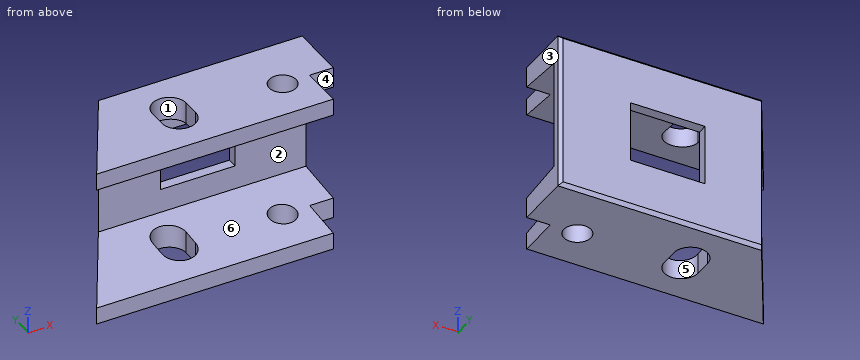
```python
from build123d import *

# Parameters (mm, degrees)
SKETCH1_R           = 4
BOSS_EXTRUDE1_DEPTH = 23.5
CUT_EXTRUDE1_REACH  = 87.914
CUT_EXTRUDE2_REACH  = 58.712
SKETCH3_W           = 22
SKETCH3_H           = 18
CHAMFER1_SIZE       = 1


with BuildPart() as part:
    # Sketch1 → Boss-Extrude1 (new, symmetric)
    with BuildSketch(Plane.XY):
        Polygon((-35, 0), (35, 0), (35, 12.5), (42, 12.5), (42, 30), (-17.679491924, 30), align=None)
        with Locations((27, 12.5)):
            Circle(SKETCH1_R, mode=Mode.SUBTRACT)
        with BuildLine():
            Line((-9, 12), (-9, 17))
            ThreePointArc((-9, 17), (-4, 22), (1, 17))
            Line((1, 17), (1, 12))
            ThreePointArc((1, 12), (-4, 7), (-9, 12))
        make_face(mode=Mode.SUBTRACT)
    extrude(amount=BOSS_EXTRUDE1_DEPTH, both=True)

    # Sketch2 → Cut-Extrude1 (cut, up to next)
    with BuildSketch(Plane(origin=(42, 0, 0), x_dir=(0, 0, -1), z_dir=(1, 0, 0)), mode=Mode.PRIVATE) as cut_extrude1_sk1:
        Polygon((-18.5, 0), (18.5, 0), (16.137806085, 27), (-16.137806085, 27), align=None)
    cut_extrude1_tool1 = extrude(cut_extrude1_sk1.sketch, amount=-CUT_EXTRUDE1_REACH, mode=Mode.PRIVATE) & part.part
    add(cut_extrude1_tool1.solids().sort_by_distance((42, 13.193114, 0))[0], mode=Mode.SUBTRACT)

    # Sketch3 → Cut-Extrude2 (cut, up to next)
    with BuildSketch(Plane(origin=(0, 30, 0), x_dir=(1, 0, 0), z_dir=(0, 1, 0)), mode=Mode.PRIVATE) as cut_extrude2_sk1:
        with Locations((10, 0)):
            Rectangle(SKETCH3_W, SKETCH3_H)
    cut_extrude2_tool1 = extrude(cut_extrude2_sk1.sketch, amount=-CUT_EXTRUDE2_REACH, mode=Mode.PRIVATE) & part.part
    add(cut_extrude2_tool1.solids().sort_by_distance((10, 30, 0))[0], mode=Mode.SUBTRACT)

    # Chamfer1
    chamfer1_edges = [part.edges().sort_by_distance(p)[0] for p in [
        (42, 30, 0),
        (12.160254038, 30, 23.5),
        (12.160254038, 30, -23.5),
    ]]
    chamfer(chamfer1_edges, length=CHAMFER1_SIZE)


solid = part.part
```
For this review, take the finished solid that the model builds, in its own axes (mm). Face numbers are marked on the shaded views. A direction names the side the tool comes from. Round coordinates to 2 decimals unless told otherwise and drop trailing zeros. Loops run counter-clockwise (first coordinate to the right, second up) from the corner with the lowest first, then second, coordinate; pieces in that order, holes last.
(1) We need section D-D (x = 27). Give the boundary of the cut face in (y, z).
Returned:
outline: (0, -23.5) - (8.5, -23.5) - (8.5, -17.76) - (0, -18.5) - close; (0, 18.5) - (8.5, 17.76) - (8.5, 23.5) - (0, 23.5) - close; (16.5, -23.5) - (29, -23.5) - (30, -22.5) - (30, 22.5) - (29, 23.5) - (16.5, 23.5) - (16.5, 17.06) - (27, 16.14) - (27, -16.14) - (16.5, -17.06) - close
(2) Mouldability with a two-part tool opening along Y and no side actions: class the marked faces 1, 2 and 3 as released by +Y, released by -Y, zero draft, split by the parting line, or undercut.
Returned:
face 1: undercut
face 2: released by -Y
face 3: zero draft
(3) Tool access review of the marked faces 4, 5 and 6: name each direction out of +Z, -Z, +X, -X, +Y, -Y from which nothing blocks a thin tool from reaching the whole face with its end or side.
Returned:
face 4: +Z, -Z, +X, -Y
face 5: +Z, -Z
face 6: +X, -X, -Y
(4) Clearance check with flat-ended pins moving along their axes: P1, Ø5, axis at x = 27, y = 12.5, coming from the +Z side; P2, Ø5.5, axis at y = 15, z = 20, coming from the -X side; P3, Ø16, axis at x = 18, z = 2.5, coming from the -Y side; P4, Ø5, axis at y = 6, z = 21.5, coming from the +X side. State where each tip first meets the part, or that it passes through.
Returned:
P1: passes through
P2: stops at x = -27.93
P3: stops at y = 27
P4: stops at x = 35
(5) Wall thickness on line 1 along Y through (x, z) = (27, 21.75); line 2 along X through (y, z) = (12, -19); line 3 along Z through (x, y) = (-15, 8.5): over which ranges is each line inside the solid? List them lowest first.
Returned:
line 1: y = 0 to 8.5, 16.5 to 30
line 2: x = -28.07 to -9, 1 to 23.03, 30.97 to 35
line 3: z = -23.5 to -17.76, 17.76 to 23.5
(6) We need section B-B (z = -4.5). Give the boundary of the cut face in (x, y), plus the area to 3 significant figures.
Returned:
outline: (-19.41, 27) - (-1, 27) - (-1, 30) - (-17.68, 30) - close; (21, 27) - (42, 27) - (42, 29) - (41, 30) - (21, 30) - close
area: 115 mm2
(7) We need section C-C (y = 24). Give the boundary of the cut face in (x, z).
Returned:
outline: (-21.14, -23.5) - (42, -23.5) - (42, -16.4) - (-21.14, -16.4) - close; (-21.14, 16.4) - (42, 16.4) - (42, 23.5) - (-21.14, 23.5) - close
(8) We need section A-A (x = 18). Give the boundary of the cut face in (y, z), plus the area to 3 significant figures.
Returned:
outline: (0, -23.5) - (29, -23.5) - (30, -22.5) - (30, -9) - (27, -9) - (27, -16.14) - (0, -18.5) - close; (0, 18.5) - (27, 16.14) - (27, 9) - (30, 9) - (30, 22.5) - (29, 23.5) - (0, 23.5) - close
area: 420 mm2
